from build123d import *

# Parameters (mm, degrees)
SKETCH1_R           = 50
SKETCH1_R_2         = 5
SKETCH1_R_3         = 7.5
SKETCH1_R_4         = 10
BOSS_EXTRUDE1_DEPTH = 5
SKETCH2_W           = 20
SKETCH2_H           = 7
BOSS_EXTRUDE2_DEPTH = 20
FILLET1_R           = 10
SKETCH3_R           = 5
CUT_EXTRUDE1_DEPTH  = 82.04221019


with BuildPart() as part:
    # Sketch1 → Boss-Extrude1 (new, symmetric)
    with BuildSketch(Plane(origin=(0, 0, 0), x_dir=(1, 0, 0), z_dir=(0, 1, 0))):
        with Locations(Location((0, 0, 0), (0, 0, 270))):
            Circle(SKETCH1_R)
        with Locations(Location((27.43826166, -17.418145627, 0), (0, 0, 270))):
            Circle(SKETCH1_R_2, mode=Mode.SUBTRACT)
        with Locations(Location((-32.5, 0, 0), (0, 0, 270))):
            Circle(SKETCH1_R_3, mode=Mode.SUBTRACT)
        with Locations(Location((0, 32.5, 0), (0, 0, 270))):
            Circle(SKETCH1_R_2, mode=Mode.SUBTRACT)
        with Locations(Location((0, 0, 0), (0, 0, 270))):
            Circle(SKETCH1_R_4, mode=Mode.SUBTRACT)
    extrude(amount=BOSS_EXTRUDE1_DEPTH, both=True)

    # Sketch2 → Boss-Extrude2 (add)
    with BuildSketch(Plane(origin=(0, 5, 0), x_dir=(1, 0, 0), z_dir=(0, 1, 0))):
        with Locations((27.570975848, 12.175717572)):
            Rectangle(SKETCH2_W, SKETCH2_H)
    extrude(amount=BOSS_EXTRUDE2_DEPTH)

    # Fillet1
    fillet1_edges = [part.edges().sort_by_distance(p)[0] for p in [
        (17.570975848, 25, -12.175717572),
        (37.570975848, 25, -12.175717572),
    ]]
    fillet(fillet1_edges, radius=FILLET1_R - 0.0001)  # a hair under: the kernel refuses the full size

    # Sketch3 → Cut-Extrude1 (cut, through all)
    with BuildSketch(Plane.XY.offset(-8.675717572)):
        with Locations((27.570975848, 15)):
            Circle(SKETCH3_R)
    extrude(amount=-CUT_EXTRUDE1_DEPTH, mode=Mode.SUBTRACT)


solid = part.part
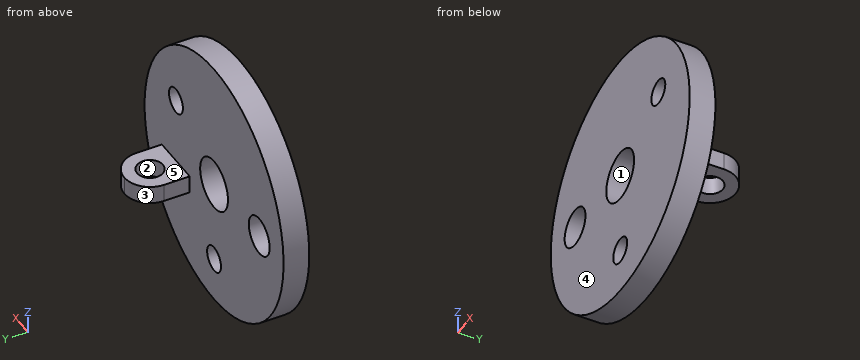
CAD build for the part. Positions are in the model's coordinates, mm. Face numbers are marked on the shaded views. A direction names the side the tool comes from. Round coordinates to 2 decimals unless told otherwise and drop trailing zeros. Order: outer loops, then holes, each group sorted by start corner. A loop starts at its lowest first (then second) coordinate and runs counter-clockwise, first axis right, second up. Notation, with made-up numbers: (6, 6.25) -> (17, 6.25) arc R25 ccw to (17, 23.25) -> close; hole circle Ø3 at (67.5, -28). An arc over 180 degrees is marked (long way). Write item = value, one per line. Start each with the question number.
(1) Pin check, flat tips, straight feed: P1, Ø12, axis at y = 0, z = 37, coming from the +X side; P2, Ø8, axis at x = 15, y = 12.5, coming from the -Z side; P3, Ø5.5, axis at y = 12, z = -12.5, coming from the +X side. Stop position of each tip, or through.
(2) Probe line 1 (X direction, y = -2.5, z = 0); line 2 (X direction, y = 4.5, z = 5.5); line 3 (Y direction, x = 9.5, z = 41). List the from-to ranges inside material, lowest first. Write a range as [from, to].
(3) Cut at A-A, the plane z = 0. List the corners of the cut face in (x, y).
(4) Cut at B-B, the plane x = 0. List the corners of the cut face in (y, z).
(5) Pull direction Y, two halves, no side cores. Call the marked faces 1, 2 and 3: released by +Y, released by -Y, zero draft, split by the parting line, or undercut.
(6) Which spindle directions (+Z, -Z, +X, -X, +Y, -Y) get a long thin tool onto all of the face, cutting with end or side? Do the marked faces 4 and 5. Say none if no direction does.
(7) Cut at C-C, the plane y = 11.5. List the corners of the cut face in (x, z).
(8) Cut at D-D, the plane z = -32.5. List the corners of the cut face in (x, y), then the cut area to 3 significant figures.
Model answer:
q1.P1 = 39.23
q1.P2 = -15.68
q1.P3 = 37.57
q2.line_1 = [-50, -40], [-25, -10], [10, 50]
q2.line_2 = [-49.7, -37.6], [-27.4, -8.35], [8.35, 49.7]
q2.line_3 = [-5, 5]
q3.outline = (-50, -5) -> (-40, -5) -> (-40, 5) -> (-50, 5) -> close; (-25, -5) -> (-10, -5) -> (-10, 5) -> (-25, 5) -> close; (10, -5) -> (50, -5) -> (50, 5) -> (10, 5) -> close
q4.outline = (-5, -50) -> (5, -50) -> (5, -37.5) -> (-5, -37.5) -> close; (-5, -27.5) -> (5, -27.5) -> (5, -10) -> (-5, -10) -> close; (-5, 10) -> (5, 10) -> (5, 50) -> (-5, 50) -> close
q5.face_1 = zero draft
q5.face_2 = undercut
q5.face_3 = released by +Y
q6.face_4 = +Z, -Z, +X, -X, -Y
q6.face_5 = +Z, +X, -X, +Y
q7.outline = (17.57, -15.68) -> (24, -15.68) -> (24, -8.68) -> (17.57, -8.68) -> close; (31.14, -15.68) -> (37.57, -15.68) -> (37.57, -8.68) -> (31.14, -8.68) -> close
q8.outline = (-38, -5) -> (-5, -5) -> (-5, 5) -> (-38, 5) -> close; (5, -5) -> (38, -5) -> (38, 5) -> (5, 5) -> close
q8.area = 660 mm2
